from build123d import *

# Parameters (mm, degrees)
SKETCH1_R           = 49
SKETCH1_R_2         = 34
BOSS_EXTRUDE1_DEPTH = 5
SKETCH2_R           = 2.55
CUT_EXTRUDE1_DEPTH  = 70.476614771


with BuildPart() as part:
    # Sketch1 → Boss-Extrude1 (new body)
    with BuildSketch(Plane.XY):
        Circle(SKETCH1_R)
        Circle(SKETCH1_R_2, mode=Mode.SUBTRACT)
    extrude(amount=BOSS_EXTRUDE1_DEPTH)

    # Sketch2 → Cut-Extrude1 (cut, through all)
    with BuildSketch(Plane.XY):
        with Locations((0, 40)):
            Circle(SKETCH2_R)
        with Locations((34.641016151, 20)):
            Circle(SKETCH2_R)
        with Locations((34.641016151, -20)):
            Circle(SKETCH2_R)
        with Locations((0, -40)):
            Circle(SKETCH2_R)
        with Locations((-34.641016151, -20)):
            Circle(SKETCH2_R)
        with Locations((-34.641016151, 20)):
            Circle(SKETCH2_R)
    extrude(amount=CUT_EXTRUDE1_DEPTH, mode=Mode.SUBTRACT)


solid = part.part
Verification items for the finished model (mm, model axes). Coordinates: 2 decimals unless noted, no trailing zeros. Order: outer loops, then holes, each group sorted by start corner. A loop starts at its lowest first (then second) coordinate and runs counter-clockwise, first axis right, second up. Notation, with made-up numbers: M 89,-16 L 117,-16 A15 cw 117,1 Z; hole C 53.25,-31.5 d8. An arc over 180 degrees is marked long. One line per item, written item: value. Start each with the question number.
Item 1: Sectioned sample at A-A (y = 0). Enter the section's corners in (x, z), then the cut area to 3 significant figures.
Item 2: Gauge pin test, flat ends, axial feed: pin 1 (2 mm diameter, centred on y = -5.5, z = 2.5, fed in from -X); pin 2 (1 mm diameter, centred on x = 36, z = 2.5, fed in from +Y) (3 decimals); pin 3 (1 mm diameter, centred on x = -39, z = 4, fed in from +Y). Record the tip position at first contact, or that the pin passes through.
Item 3: Sectioned sample at D-D (y = -20). Enter the section's corners in (x, z).
Item 4: Scan lines: probe 1 along Y at (x, z) = (0, 3.2); probe 2 along X at (y, z) = (-18, 4.3); probe 3 along Y at (x, z) = (35.5, 3.7) (3 decimals). Record each from-to range of solid material in increasing order.
Item 5: Sectioned sample at C-C (x = 0). Enter the section's corners in (y, z), then the cut area to 3 significant figures.
Item 6: Sectioned sample at B-B (z = 3.75). Enter the section's corners in (x, y), then the cut area to 3 significant figures.
Item 7: Mould release check, pull along Y, two halves, no side actions. Record for faces 1 (the flat face through (32, 12, 5)), 2 (the cylindrical face through (-0.33, -37.47, 2.46)), 3 (the cylindrical face through (26.34, 41.32, 2.46)): released by +Y, released by -Y, zero draft, split by the parting line, or undercut.
Conclusion:
1. outline: M -49,0 L -34,0 L -34,5 L -49,5 Z; M 34,0 L 49,0 L 49,5 L 34,5 Z
1. area: 150 mm^2
2. pin 1: stops at x = -48.79
2. pin 2: stops at y = 33.775
2. pin 3: stops at y = 30.31
3. outline: M -44.73,0 L -37.19,0 L -37.19,5 L -44.73,5 Z; M -32.09,0 L -27.5,0 L -27.5,5 L -32.09,5 Z; M 27.5,0 L 32.09,0 L 32.09,5 L 27.5,5 Z; M 37.19,0 L 44.73,0 L 44.73,5 L 37.19,5 Z
4. probe 1: y = -49 to -42.55, -37.45 to -34, 34 to 37.45, 42.55 to 49
4. probe 2: x = -45.57 to -36.22, -33.06 to -28.84, 28.84 to 33.06, 36.22 to 45.57
4. probe 3: y = -33.775 to -22.401, -17.599 to 17.599, 22.401 to 33.775
5. outline: M -49,0 L -42.55,0 L -42.55,5 L -49,5 Z; M -37.45,0 L -34,0 L -34,5 L -37.45,5 Z; M 34,0 L 37.45,0 L 37.45,5 L 34,5 Z; M 42.55,0 L 49,0 L 49,5 L 42.55,5 Z
5. area: 99.0 mm^2
6. outline: C 0,0 d98; hole C -34.64,-20 d5.1; hole C -34.64,20 d5.1; hole C 0,0 d68; hole C 0,-40 d5.1; hole C 0,40 d5.1; hole C 34.64,-20 d5.1; hole C 34.64,20 d5.1
6. area: 3,790 mm^2
7. face 1: zero draft
7. face 2: undercut
7. face 3: split by the parting line
